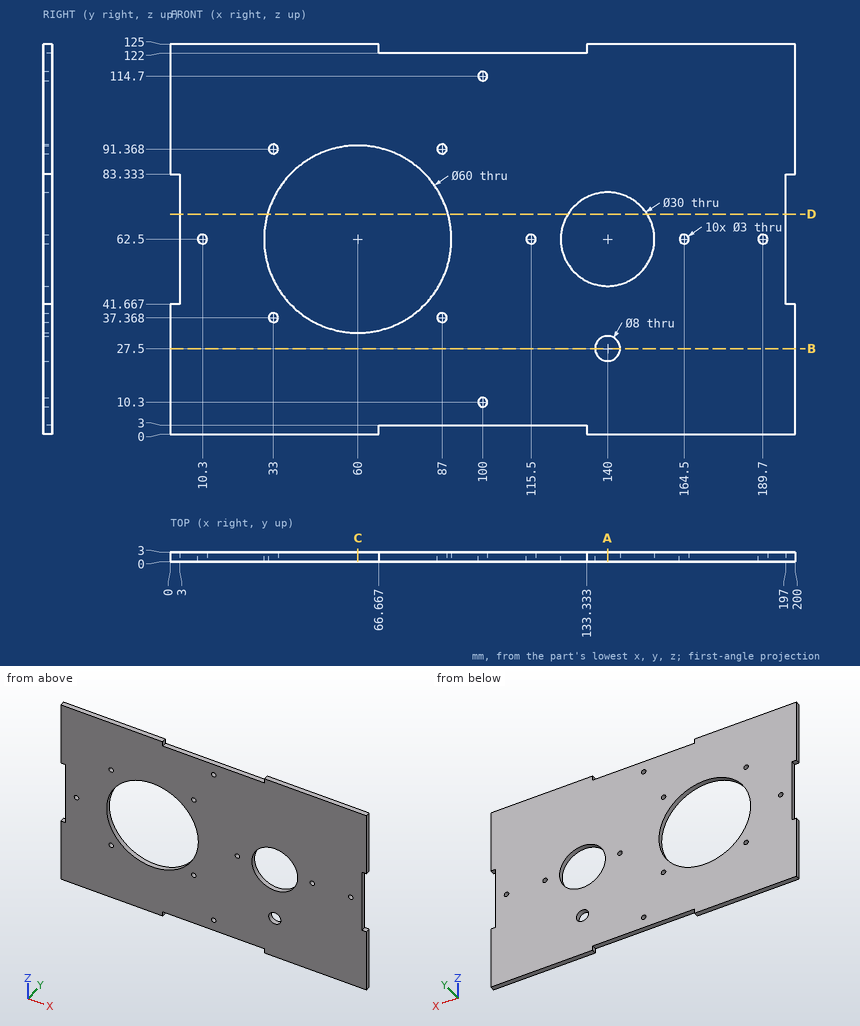
Source: three-view drawing plus pictorial views. Frame: mm from the lowest corner of the part. Coordinates: 2 decimals unless noted, no trailing zeros. Loops run counter-clockwise (first coordinate to the right, second up) from the corner with the lowest first, then second, coordinate; pieces in that order, holes last. Notation, with made-up numbers: (-25, 84) -> (34, 84) arc R19 ccw to (34, 115) -> close; hole circle Ø2 at (-27.75, 63). An arc over 180 degrees is marked (long way). One line per item, written item: value.
(1) Ray query, line 1 along Z through (x, y) = (10.3, 2.25); line 2 along Z through (x, y) = (140, 1.65); line 3 along Z through (x, y) = (115.5, 2.1). Return the intervals inside material, ascending.
Answer below:
line 1: z = 0 to 61, 64 to 125
line 2: z = 0 to 23.5, 31.5 to 47.5, 77.5 to 125
line 3: z = 3 to 61, 64 to 122
(2) Cut plane D-D (z = 70.5). Output: boundary loops of the cut face in (x, y).
Answer below:
outline: (3, 0) -> (31.09, 0) -> (31.09, 3) -> (3, 3) -> close; (88.91, 0) -> (127.31, 0) -> (127.31, 3) -> (88.91, 3) -> close; (152.69, 0) -> (197, 0) -> (197, 3) -> (152.69, 3) -> close
(3) Pin query (flat end, axial travel): pin 1 Ø6 at (x, z) = (43.5, 103.5) entering from -Y; pin 2 Ø6.5 at (x, z) = (140, 27.5) entering from +Y; pin 3 Ø1.5 at (y, z) = (1, 71) entering from -X; pin 4 Ø0.9 at (y, z) = (2, 52) entering from +X. Return the tip coordinate at first contact, or that it passes through.
Answer below:
pin 1: stops at y = 0
pin 2: passes through
pin 3: stops at x = 3
pin 4: stops at x = 197
(4) Cut plane B-B (z = 27.5). Output: boundary loops of the cut face in (x, y), then the cut area to 3 significant figures.
Answer below:
outline: (0, 0) -> (136, 0) -> (136, 3) -> (0, 3) -> close; (144, 0) -> (200, 0) -> (200, 3) -> (144, 3) -> close
area: 576 mm2
(5) Cut plane A-A (x = 140). Output: boundary loops of the cut face in (y, z).
Answer below:
outline: (0, 0) -> (3, 0) -> (3, 23.5) -> (0, 23.5) -> close; (0, 31.5) -> (3, 31.5) -> (3, 47.5) -> (0, 47.5) -> close; (0, 77.5) -> (3, 77.5) -> (3, 125) -> (0, 125) -> close
(6) Cut plane C-C (x = 60). Output: boundary loops of the cut face in (y, z), then the cut area to 3 significant figures.
Answer below:
outline: (0, 0) -> (3, 0) -> (3, 32.5) -> (0, 32.5) -> close; (0, 92.5) -> (3, 92.5) -> (3, 125) -> (0, 125) -> close
area: 195 mm2
